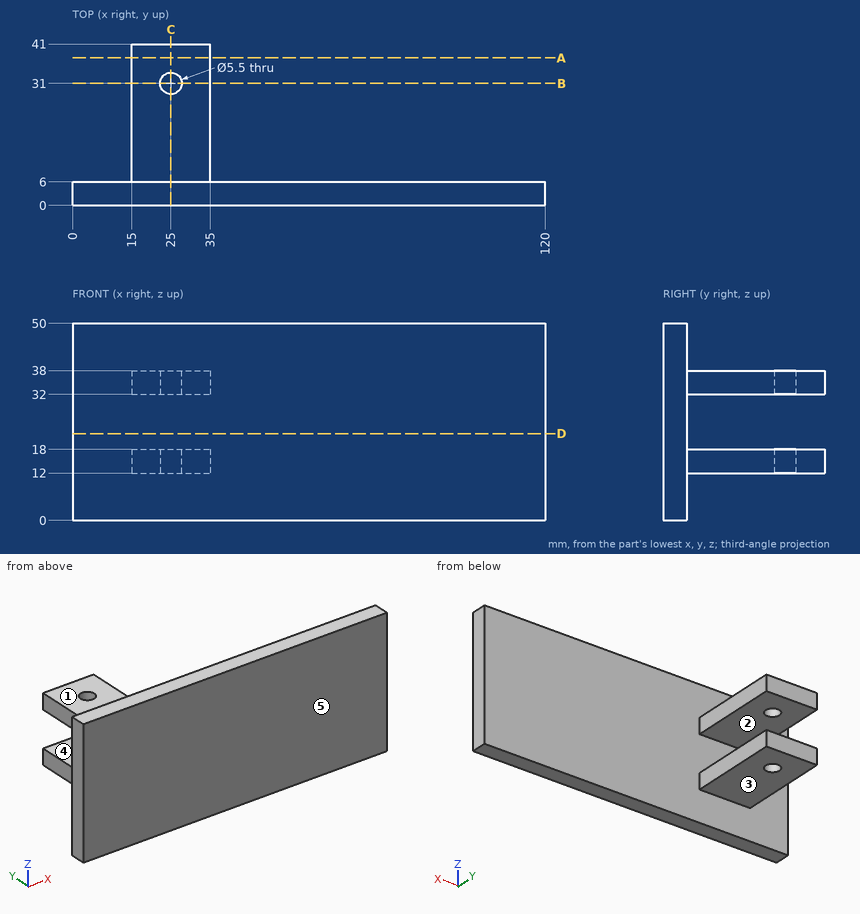
Study the drawing (mm; zero at the part's minimum x, y, z) and answer. A direction names the side the tool comes from. Round coordinates to 2 decimals unless told otherwise and drop trailing zeros. Loops run counter-clockwise (first coordinate to the right, second up) from the corner with the lowest first, then second, coordinate; pieces in that order, holes last. Notation, with made-up numbers: (-36.75, 11) -> (-1.75, 11) arc R9 cw to (-1.75, 15) -> close; hole circle Ø11 at (81, -23.75). An arc over 180 degrees is marked (long way). One line per item, written item: value.
1) A cutting plane is placed at B-B (y = 31). Determine the outline of the cut face in (x, z).
Answer list:
outline: (15, 12) -> (22.25, 12) -> (22.25, 18) -> (15, 18) -> close; (15, 32) -> (22.25, 32) -> (22.25, 38) -> (15, 38) -> close; (27.75, 12) -> (35, 12) -> (35, 18) -> (27.75, 18) -> close; (27.75, 32) -> (35, 32) -> (35, 38) -> (27.75, 38) -> close
2) Flat-ended cylindrical pins translate along their axes: P1, Ø10, axis at y = 24, z = 21, coming from the -X side; P2, Ø16, axis at x = 28.5, y = 23.5, coming from the +Z side; P3, Ø2, axis at x = 104.5, z = 17, coming from the +Y side. Find the tip coordinate at first contact, or state that the pin passes through.
Answer list:
P1: stops at x = 15
P2: stops at z = 38
P3: stops at y = 6
3) A cutting plane is placed at D-D (z = 22). Determine the outline of the cut face in (x, y).
Answer list:
outline: (0, 0) -> (120, 0) -> (120, 6) -> (0, 6) -> close
4) Consider L1, parallel to Y at x = 25, z = 34; L2, parallel to X at y = 31, z = 35.4; L3, parallel to Z at x = 21.5, y = 18. Determine where each line is inside the solid, lowest interval first. Write a range as [from, to].
Answer list:
L1: y = [0, 28.25], [33.75, 41]
L2: x = [15, 22.25], [27.75, 35]
L3: z = [12, 18], [32, 38]
5) For the marked faces 4 and 5, determine the directions among +Z, -Z, +X, -X, +Y, -Y from which every point of the face is accessible in a straight line to the end or side of a thin tool.
Answer list:
face 4: +X, -X, +Y
face 5: +Z, -Z, +X, -X, -Y
6) A cutting plane is placed at A-A (y = 37.5). Determine the outline of the cut face in (x, z).
Answer list:
outline: (15, 12) -> (35, 12) -> (35, 18) -> (15, 18) -> close; (15, 32) -> (35, 32) -> (35, 38) -> (15, 38) -> close
7) The mould has two halves that part along Z. Classify the marked faces 1, 2 and 3: pulls with the +Z half, pulls with the -Z half, needs draft (parallel to the pull), parting line crosses it, or undercut.
Answer list:
face 1: pulls with the +Z half
face 2: undercut
face 3: pulls with the -Z half
8) A cutting plane is placed at C-C (x = 25). Determine the outline of the cut face in (y, z).
Answer list:
outline: (0, 0) -> (6, 0) -> (6, 12) -> (28.25, 12) -> (28.25, 18) -> (6, 18) -> (6, 32) -> (28.25, 32) -> (28.25, 38) -> (6, 38) -> (6, 50) -> (0, 50) -> close; (33.75, 12) -> (41, 12) -> (41, 18) -> (33.75, 18) -> close; (33.75, 32) -> (41, 32) -> (41, 38) -> (33.75, 38) -> close
